from build123d import *

# Parameters (mm, degrees)
F1_DEPTH = 63.5
F0_W     = 25.4
F0_H     = 19.05
F2_DEPTH = 25.4


with BuildPart() as f1:
    # F0 (on Front) → F1 (new body, symmetric)
    with BuildSketch(Plane.XZ):
        Polygon((41.275, -9.525), (41.275, 9.525), (22.225, 9.525), (-41.275, 9.525), (-41.275, -9.525), align=None)
    extrude(amount=F1_DEPTH, both=True)

    # F0 (on Front) → F2 (join, symmetric)
    with BuildSketch(Plane.XZ):
        with BuildLine():
            Line((22.225, 9.525), (41.275, 9.525))
            Line((41.275, 9.525), (41.275, 26.9875))
            ThreePointArc((41.275, 26.9875), (45.92468, 38.21282), (57.15, 42.8625))
            Line((57.15, 42.8625), (60.325, 42.8625))
            Line((60.325, 42.8625), (60.325, 61.9125))
            Line((60.325, 61.9125), (57.15, 61.9125))
            ThreePointArc((57.15, 61.9125), (32.454296, 51.683204), (22.225, 26.9875))
            Line((22.225, 26.9875), (22.225, 9.525))
        make_face()
        with Locations((73.025, 52.3875)):
            Rectangle(F0_W, F0_H)
    extrude(amount=F2_DEPTH, both=True)


solid = f1.part
Work out the finished part from the listing and answer in its coordinate system (mm). A direction names the side the tool comes from. Give positions to 0.01 mm unless a question says otherwise; leave off trailing zeros. Order: outer loops, then holes, each group sorted by start corner. A loop starts at its lowest first (then second) coordinate and runs counter-clockwise, first axis right, second up. Notation, with made-up numbers: (64, 89.5) -> (79, 89.5) arc R14 ccw to (79, 104.5) -> close; hole circle Ø2 at (-32, 35). An arc over 180 degrees is marked (long way). Answer as a JSON object with one key per item and string values. Group by question number.
1. Consider line 1 along Y through (x, z) = (53.5, 53.5); line 2 along X through (y, z) = (28, 6.5) (3 decimals); line 3 along Z through (x, y) = (4, 34) (3 decimals). Determine where each line is inside the solid, lowest interval first. Write a range as [from, to].
2. Flat-ended cylindrical pins translate along their axes: pin 1 Ø5 at (y, z) = (-4, 16) entering from -X (3 decimals); pin 2 Ø11 at (y, z) = (-26.5, 5) entering from +X (3 decimals); pin 3 Ø3 at (x, y) = (43, 1.5) entering from +Z; pin 4 Ø12 at (x, y) = (61, 32.5) entering from -Z. Find the tip coordinate at first contact, or state that the pin passes through.
3. Section C-C on z = 7 is taken. Determine the outline of the cut face in (x, y) (3 decimals).
4. Section D-D on x = 34.5 is taken. Determine the outline of the cut face in (y, z) (3 decimals).
5. A tool of negligible diameter and unlimited length cuts with its end or side. For faces 1 (the flat face through (71, 0, 42.862)), 2 (the flat face through (46, -25.4, 42)), 3 (the flat face through (46, 25.4, 42)), 4 (the flat face through (22.225, 0, 18)), from which of +Z, -Z, +X, -X, +Y, -Y can it reach the whole face along a straight path? Write none if from no direction.
6. Section B-B on x = 71 is taken. Determine the outline of the cut face in (y, z), plus the area to 3 significant figures.
Result sheet:
{
 "1": {"line 1": "y = [-25.4, 25.4]", "line 2": "x = [-41.275, 41.275]", "line 3": "z = [-9.525, 9.525]"},
 "2": {"pin 1": "stops at x = 22.225", "pin 2": "stops at x = 41.275", "pin 3": "stops at z = 59.54", "pin 4": "passes through"},
 "3": {"outline": "(-41.275, -63.5) -> (41.275, -63.5) -> (41.275, 63.5) -> (-41.275, 63.5) -> close"},
 "4": {"outline": "(-63.5, -9.525) -> (63.5, -9.525) -> (63.5, 9.525) -> (25.4, 9.525) -> (25.4, 53.572) -> (-25.4, 53.572) -> (-25.4, 9.525) -> (-63.5, 9.525) -> close"},
 "5": {"face 1": "-Z, +X, +Y, -Y", "face 2": "+Z, +X, -X, -Y", "face 3": "+Z, +X, -X, +Y", "face 4": "+Z, -X, +Y, -Y"},
 "6": {"outline": "(-25.4, 42.86) -> (25.4, 42.86) -> (25.4, 61.91) -> (-25.4, 61.91) -> close", "area": "968 mm^2"}
}
